```python
from build123d import *

# Parameters (mm, degrees)
ESQUISSE1_W        = 23.5
ESQUISSE1_H        = 20.5
CORPS_DEPTH        = 6.1
COQUE1_T           = 2
PIVOT_SORTIE_DEPTH = 24.5
ESQUISSE3_R        = 1.875
AXE_SORTIE_DEPTH   = 3
ESQUISSE4_W        = 31.6
ESQUISSE4_H        = 12.2
ESQUISSE4_R        = 1
MIP_MAP_DEPTH      = 1.5
CONG_1_R           = 3
CONG_2_R           = 0.5


with BuildPart() as part:
    # Esquisse1 → corps (new body, symmetric)
    with BuildSketch(Plane.XY):
        with Locations((0, 10.25)):
            Rectangle(ESQUISSE1_W, ESQUISSE1_H)
    extrude(amount=CORPS_DEPTH, both=True)

    # Coque1 (no face opened: a closed hollow body)
    add(offset(amount=-COQUE1_T, mode=Mode.PRIVATE), mode=Mode.SUBTRACT)

    # Esquisse2 → pivot_sortie (add)
    with BuildSketch(Plane(origin=(0, 0, 0), x_dir=(1, 0, 0), z_dir=(0, 1, 0))):
        with BuildLine():
            ThreePointArc((-2.125, 3.443744328), (-10.75, 0), (-2.125, -3.443744328))
            ThreePointArc((-2.125, -3.443744328), (-0.876409356, -2.488320716), (0.607142857, -1.967853902))
            ThreePointArc((0.607142857, -1.967853902), (2.25, 0), (0.607142857, 1.967853902))
            ThreePointArc((0.607142857, 1.967853902), (-0.876409356, 2.488320716), (-2.125, 3.443744328))
        make_face()
    extrude(amount=PIVOT_SORTIE_DEPTH)

    # Esquisse3 → axe_sortie (add)
    with BuildSketch(Plane(origin=(0, 24.5, 0), x_dir=(1, 0, 0), z_dir=(0, 1, 0))):
        with Locations((-5.75, 0)):
            Circle(ESQUISSE3_R)
    extrude(amount=AXE_SORTIE_DEPTH)

    # Esquisse4 → MIP_MAP (add)
    with BuildSketch(Plane.XZ.offset(-15)):
        Rectangle(ESQUISSE4_W, ESQUISSE4_H)
        with Locations((-13.8, 0)):
            Circle(ESQUISSE4_R, mode=Mode.SUBTRACT)
        with Locations((13.8, 0)):
            Circle(ESQUISSE4_R, mode=Mode.SUBTRACT)
    extrude(amount=-MIP_MAP_DEPTH)

    # Congé1
    cong_1_edges = [part.edges().sort_by_distance(p)[0] for p in [
        (15.8, 15.75, -6.1),
        (-15.8, 15.75, 6.1),
        (15.8, 15.75, 6.1),
        (-15.8, 15.75, -6.1),
    ]]
    fillet(cong_1_edges, radius=CONG_1_R)

    # Congé2
    cong_2_edges = [part.edges().sort_by_distance(p)[0] for p in [
        (11.75, 7.5, 6.1),
        (0, 20.5, 6.1),
        (-11.75, 18.5, 6.1),
        (0, 20.5, -6.1),
        (11.75, 7.5, -6.1),
        (0, 0, -6.1),
        (-11.75, 18.5, -6.1),
        (0, 0, 6.1),
        (-11.75, 20.5, 0),
        (11.75, 20.5, 0),
        (11.75, 0, 0),
        (-11.75, 0, 0),
        (-11.75, 7.5, -6.1),
        (11.75, 18.5, -6.1),
        (-11.75, 7.5, 6.1),
        (11.75, 18.5, 6.1),
    ]]
    fillet(cong_2_edges, radius=CONG_2_R)


solid = part.part
```
The model under review builds one solid part; all positions refer to its coordinate system, in mm. A direction names the side the tool comes from. Coordinates: 2 decimals unless noted, no trailing zeros. Order: outer loops, then holes, each group sorted by start corner. A loop starts at its lowest first (then second) coordinate and runs counter-clockwise, first axis right, second up. Notation, with made-up numbers: (-11.5, 19) -> (14.5, 19) arc R27 cw to (14.5, 38) -> close; hole circle Ø3 at (11, -19.5). An arc over 180 degrees is marked (long way). Answer in a Markdown table with one row per item. Add a question column.
Item 1: To check wall thickness, follow probe 1 along Y at (x, z) = (9.5, -3.25); probe 2 along X at (y, z) = (5.5, 3.25); probe 3 along Z at (x, y) = (1, 8.5). State the ranges of each line that lie inside material, in increasing order.
Item 2: Clearance check with flat-ended pins moving along their axes: pin 1 (5.5 mm diameter, centred on y = 8.5, z = -2, fed in from -X); pin 2 (1.4 mm diameter, centred on x = 14, z = -3, fed in from +Y); pin 3 (0.6 mm diameter, centred on x = -9, z = -3.5, fed in from +Y). State where each tip first meets the part, or that it passes through.
Item 3: We need section C-C on x = 13.8. Write out the cut boundary in (y, z).
Item 4: Mouldability with a two-part tool opening along Y and no side actions: class faces 5 (the flat face through (-11.75, 8, 0)), 6 (the flat face through (12, 15, 0)), 7 (the flat face through (-9.4, 15, -3.8)) as +Y half, -Y half, draft (parallel to the pull), parting line (faces both ways), or undercut.
Item 5: Machinability: for faces 1 (the flat face through (-11.75, 18, 0)), 2 (the cylindrical face through (-7.623, 25.979, -0.082)), 3 (the cylindrical face through (2.25, 17.49, 0.04)), 4 (the flat face through (0, 0, 0)), which of the approach directions +Z, -Z, +X, -X, +Y, -Y give a long, thin tool a straight path to every point of the face, cutting with its end or side? Answer none if there is none.
Item 6: We need section A-A on y = 8.25. Write out the cut boundary in (x, z) (3 decimals), plus the area to 3 significant figures.
Item 7: We need section B-B on z = 0. Give the number of separate pieces and of enclosed holes in the cut face, plus the area to 3 significant figures.
Item 8: We need section D-D on x = -5.75. Write out the cut boundary in (y, z) (3 decimals).
Final values:
| question | item | result |
|---|---|---|
| 1 | probe 1 | y = 0 to 2, 15 to 16.5, 18.5 to 20.5 |
| 1 | probe 2 | x = -11.75 to -9.75, -9.55 to -1.93, 9.75 to 11.75 |
| 1 | probe 3 | z = -6.1 to -4.1, -1.85 to 1.85, 4.1 to 6.1 |
| 2 | pin 1 | stops at x = -11.75 |
| 2 | pin 2 | stops at y = 16.5 |
| 2 | pin 3 | stops at y = 24.5 |
| 3 | outline | (15, -5.93) -> (16.5, -5.93) -> (16.5, -1) -> (15, -1) -> close; (15, 1) -> (16.5, 1) -> (16.5, 5.93) -> (15, 5.93) -> close |
| 4 | face 5 | draft |
| 4 | face 6 | -Y half |
| 4 | face 7 | undercut |
| 5 | face 1 | +Z, -Z, -X, +Y |
| 5 | face 2 | +Y |
| 5 | face 3 | none |
| 5 | face 4 | +Z, -Z, +X, -X, -Y |
| 6 | outline | (-11.75, -5.6) arc R0.5 ccw to (-11.25, -6.1) -> (11.25, -6.1) arc R0.5 ccw to (11.75, -5.6) -> (11.75, 5.6) arc R0.5 ccw to (11.25, 6.1) -> (-11.25, 6.1) arc R0.5 ccw to (-11.75, 5.6) -> close; hole (-9.75, -4.1) -> (-8.612, -4.1) arc R5 cw to (-9.75, -3) -> close; hole (-9.75, 3) arc R5 cw to (-8.612, 4.1) -> (-9.75, 4.1) -> close; hole (-2.888, -4.1) -> (9.75, -4.1) -> (9.75, 4.1) -> (-2.888, 4.1) arc R5 cw to (-2.125, 3.444) arc R5 ccw to (0.607, 1.968) arc R2 cw to (0.607, -1.968) arc R5 ccw to (-2.125, -3.444) arc R5 cw to start |
| 6 | area | 206 mm2 |
| 7 | separate pieces | 3 |
| 7 | enclosed holes | 2 |
| 7 | area | 438 mm2 |
| 8 | outline | (0, -5.6) arc R0.5 ccw to (0.5, -6.1) -> (20, -6.1) arc R0.5 ccw to (20.5, -5.6) -> (20.5, -5) -> (24.5, -5) -> (24.5, -1.875) -> (27.5, -1.875) -> (27.5, 1.875) -> (24.5, 1.875) -> (24.5, 5) -> (20.5, 5) -> (20.5, 5.6) arc R0.5 ccw to (20, 6.1) -> (0.5, 6.1) arc R0.5 ccw to (0, 5.6) -> close |
